```python
from build123d import *

# Parameters (mm, degrees)
F0_W     = 72
F0_H     = 20
F1_DEPTH = 10
F2_W     = 12
F2_H     = 20
F3_DEPTH = 5
F4_R     = 3
F4_R_2   = 2.1
F5_DEPTH = 25


with BuildPart() as f1:
    # F0 (on Top) → F1 (new body)
    with BuildSketch(Plane.XY):
        with Locations((36, 10)):
            Rectangle(F0_W, F0_H)
    extrude(amount=F1_DEPTH)

    # F2 (on face) → F3 (cut)
    with BuildSketch(Plane.XY.offset(10)):
        with Locations((36, 10)):
            Rectangle(F2_W, F2_H)
    extrude(amount=-F3_DEPTH, mode=Mode.SUBTRACT)

    # F4 (on face) → F5 (cut)
    with BuildSketch(Plane.XY.offset(10)):
        with Locations((6, 10)):
            Circle(F4_R)
        with Locations((66, 10)):
            Circle(F4_R)
        with Locations((36, 10)):
            Circle(F4_R_2)
    extrude(amount=-F5_DEPTH, mode=Mode.SUBTRACT)


solid = f1.part
```
Could you check a few things on this model? Use its own coordinates, in mm. A direction names the side the tool comes from. Round coordinates to 2 decimals unless told otherwise and drop trailing zeros. Order: outer loops, then holes, each group sorted by start corner. A loop starts at its lowest first (then second) coordinate and runs counter-clockwise, first axis right, second up. Notation, with made-up numbers: M 3,63.5 L 28,63.5 A22 ccw 28,88.5 Z; hole C 69,45.25 d8. An arc over 180 degrees is marked long. One line per question, with ' | ' between items. Start each with the question number.
(1) Please list where these lines run through material, in increasing order: line 1 along Y through (x, z) = (66, 7.75); line 2 along X through (y, z) = (5, 6.75); line 3 along X through (y, z) = (10.5, 5.5).
(2) Suppose I cut it at D-D on y = 10. List the corners of the cut face in (x, z) for me, then the cut area to 3 significant figures.
(3) Thinking about a two-plate mould opening in Y: for faces 3 (the face through (35, 20, 4)), 4 (the face through (35.5, 12.4, 0)), 5 (the face through (33.9, 10.09, 2.54)), which applies, +Y half, -Y half, draft (parallel to the pull), parting line (faces both ways), or undercut?
(4) Suppose I cut it at A-A on z = 8.5. List the corners of the cut face in (x, y) for me, then the cut area to 3 significant figures.
(5) Suppose I cut it at C-C on z = 4. List the corners of the cut face in (x, y) for me, then the cut area to 3 significant figures.
(6) For faces 1 (the face through (35.9, 12.4, 5)), 2 (the face through (35, 0, 4)), which set-ups out of +Z, -Z, +X, -X, +Y, -Y let a thin tool reach every point of the face, with its end or its side?
(7) Suppose I cut it at B-B on x = 66. List the corners of the cut face in (y, z) for me.
Geometry results:
1) line 1: 0 to 7, 13 to 20 | line 2: 0 to 30, 42 to 72 | line 3: 0 to 3.04, 8.96 to 30, 42 to 63.04, 68.96 to 72
2) outline: M 0,0 L 3,0 L 3,10 L 0,10 Z; M 9,0 L 33.9,0 L 33.9,5 L 30,5 L 30,10 L 9,10 Z; M 38.1,0 L 63,0 L 63,10 L 42,10 L 42,5 L 38.1,5 Z; M 69,0 L 72,0 L 72,10 L 69,10 Z | area: 519 mm²
3) face 3: +Y half | face 4: draft | face 5: undercut
4) outline: M 0,0 L 30,0 L 30,20 L 0,20 Z; M 42,0 L 72,0 L 72,20 L 42,20 Z; hole C 6,10 d6; hole C 66,10 d6 | area: 1,140 mm²
5) outline: M 0,0 L 72,0 L 72,20 L 0,20 Z; hole C 6,10 d6; hole C 36,10 d4.2; hole C 66,10 d6 | area: 1,370 mm²
6) face 1: +Z, +Y, -Y | face 2: +Z, -Z, +X, -X, -Y
7) outline: M 0,0 L 7,0 L 7,10 L 0,10 Z; M 13,0 L 20,0 L 20,10 L 13,10 Z
